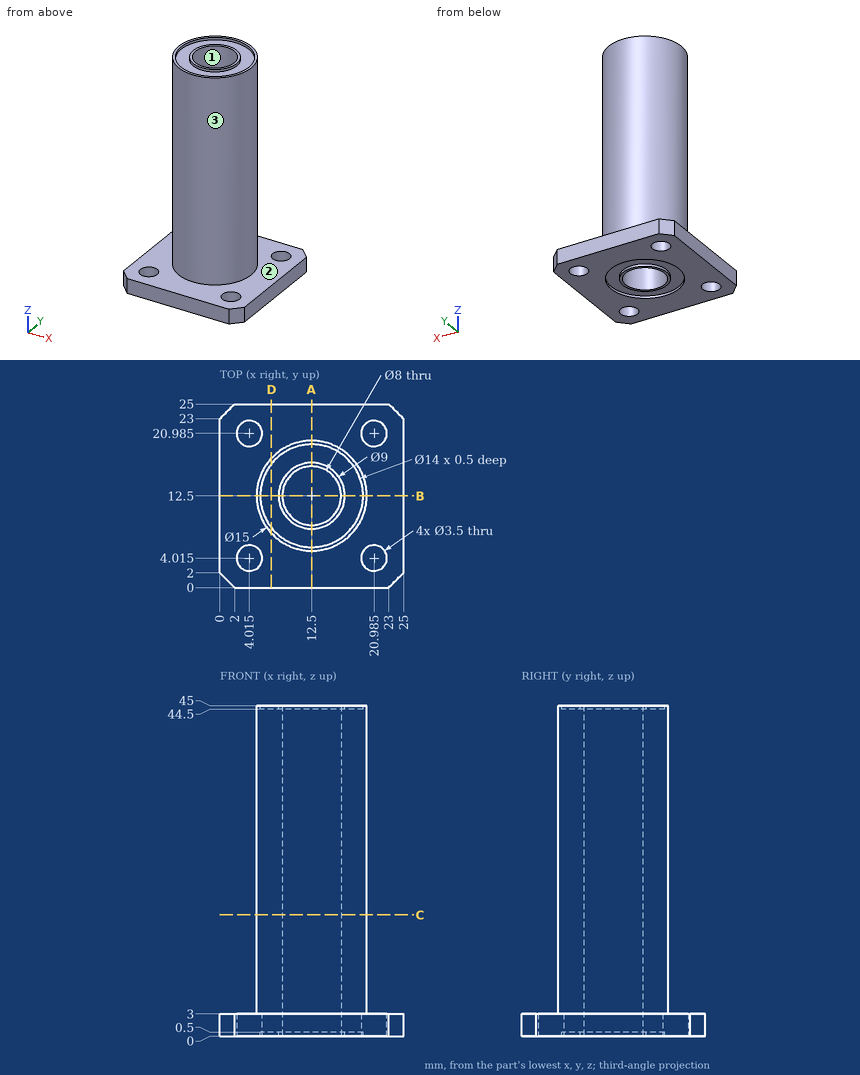
Could you check a few things on this drawing? It's one solid part, dimensions in mm from its lowest x, y, z. Give positions to 0.01 mm unless a question says otherwise; leave off trailing zeros. Write each loop counter-clockwise with the first axis right and the second up, starting at its lowest first coordinate (ties: lowest second). Pieces come first, ordered by that corner, then holes. Notation, with made-up numbers: (28, -21.75) -> (72, -21.75) arc R23 ccw to (72, 6.25) -> close; hole circle Ø11 at (68.25, 28). An arc over 180 degrees is marked (long way). Answer as a JSON object with one key per item and string values.
Q1. Suppose I cut it at D-D on x = 7. Write out the boundary of the cut face in (y, z).
Taken from the geometry:
{"outline": "(0, 0) -> (8.17, 0) -> (8.17, 0.5) -> (16.83, 0.5) -> (16.83, 0) -> (25, 0) -> (25, 3) -> (17.6, 3) -> (17.6, 45) -> (16.83, 45) -> (16.83, 44.5) -> (8.17, 44.5) -> (8.17, 45) -> (7.4, 45) -> (7.4, 3) -> (0, 3) -> close"}
Q2. We'd pull the mould along Y, two halves only. Please class the marked faces 1, 2 and 3: released by +Y, released by -Y, zero draft, split by the parting line, or undercut.
Taken from the geometry:
{"face 1": "undercut", "face 2": "zero draft", "face 3": "split by the parting line"}
Q3. Suppose I cut it at A-A on x = 12.5. Write out the boundary of the cut face in (y, z).
Taken from the geometry:
{"outline": "(0, 0) -> (5.5, 0) -> (5.5, 0.5) -> (8, 0.5) -> (8, 0) -> (8.5, 0) -> (8.5, 45) -> (8, 45) -> (8, 44.5) -> (5.5, 44.5) -> (5.5, 45) -> (5, 45) -> (5, 3) -> (0, 3) -> close; (16.5, 0) -> (17, 0) -> (17, 0.5) -> (19.5, 0.5) -> (19.5, 0) -> (25, 0) -> (25, 3) -> (20, 3) -> (20, 45) -> (19.5, 45) -> (19.5, 44.5) -> (17, 44.5) -> (17, 45) -> (16.5, 45) -> close"}
Q4. Suppose I cut it at C-C on z = 16.5. Write out the boundary of the cut face in (x, y), then the cut area to 3 significant figures.
Taken from the geometry:
{"outline": "circle Ø15 at (12.5, 12.5); hole circle Ø8 at (12.5, 12.5)", "area": "126 mm²"}
Q5. Will these pins go through, and if not, where does the flat tip stop? pin 1 Ø4 at (x, z) = (14, 33) entering from -Y; pin 2 Ø2 at (y, z) = (13.5, 15) entering from -X; pin 3 Ø3 at (x, z) = (18, 37) entering from +Y (1 decimal).
Taken from the geometry:
{"pin 1": "stops at y = 5", "pin 2": "stops at x = 5", "pin 3": "stops at y = 18.8"}
Q6. Please list where these lines run through material, in increasing order: L1, parallel to Y at x = 12.5, z = 0.2; L2, parallel to Z at x = 4.75, y = 18.75; L3, parallel to Z at x = 5.75, y = 11.75.
Taken from the geometry:
{"L1": "y = 0 to 5.5, 8 to 8.5, 16.5 to 17, 19.5 to 25", "L2": "z = 0 to 3", "L3": "z = 0.5 to 44.5"}
